For this review, use the dimensioned drawing (mm, ordinates from the lowest corner) and the shaded views. Coordinates: 2 decimals unless noted, no trailing zeros. Loops run counter-clockwise (first coordinate to the right, second up) from the corner with the lowest first, then second, coordinate; pieces in that order, holes last. Notation, with made-up numbers: (86, 82) - (100, 82) arc R28 cw to (100, 112) - close; hole circle Ø4 at (20.25, 70). An arc over 180 degrees is marked (long way). Answer in a Markdown table with one row per item. Add a question column.
(1) We need section B-B, the plane z = 22.5. Write out the cut boundary in (x, y), plus the area to 3 significant figures.
(2) To check wall thickness, follow L1, parallel to Y at x = 24, z = 10.5; L2, parallel to Y at x = 23.5, z = 1.5; L3, parallel to Z at x = 11.5, y = 41. State the ranges of each line that lie inside material, in increasing order. Write a range as [from, to].
(3) Clearance check with flat-ended pins moving along their axes: pin 1 (9 mm diameter, centred on x = 24, y = 24, fed in from -Z); pin 2 (1.5 mm diameter, centred on x = 18.5, z = 4.5, fed in from +Y); pin 3 (5 mm diameter, centred on y = 13, z = 13, fed in from -X); pin 4 (3 mm diameter, centred on x = 31.5, z = 7, fed in from +Y). State where each tip first meets the part, or that it passes through.
(4) The part is to be moulded in two halves that separate along Y. For the marked faces 1, 2 and 3, say which applies: released by +Y, released by -Y, zero draft, split by the parting line, or undercut.
(5) We need section A-A, the plane z = 6.25. Write out the cut boundary in (x, y).
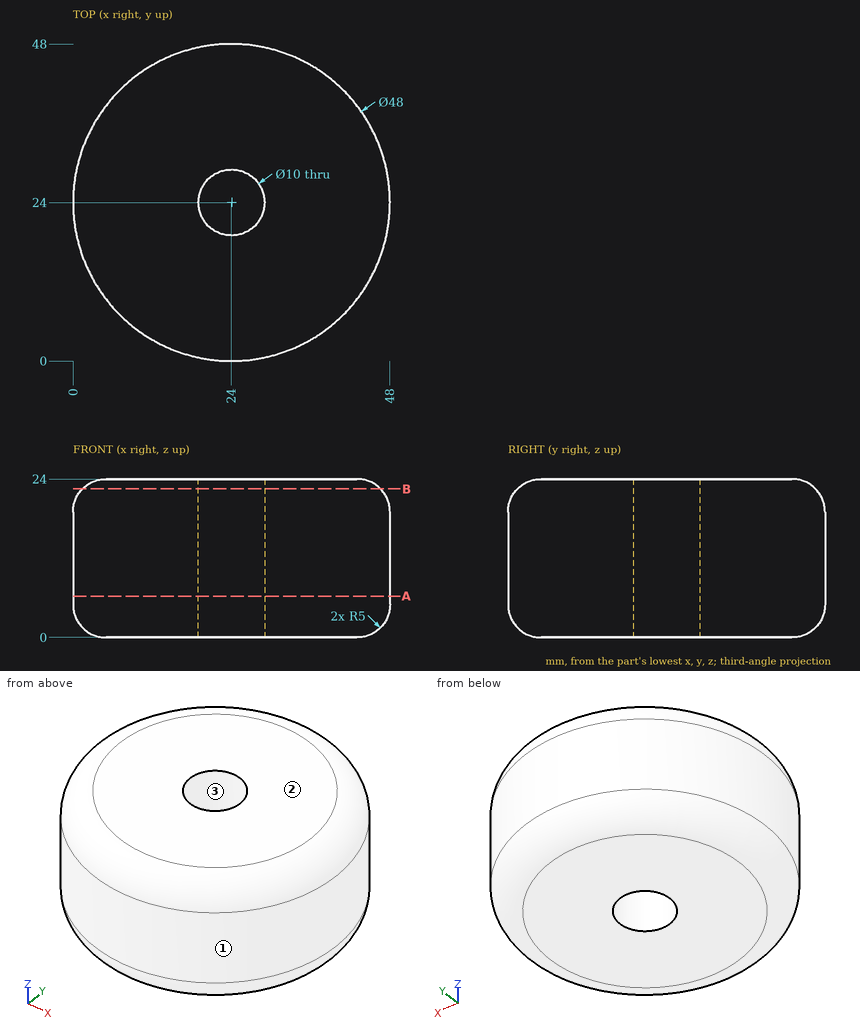
Responses:
| question | item | result |
|---|---|---|
| 1 | outline | circle Ø45.14 at (24, 24); hole circle Ø10 at (24, 24) |
| 1 | area | 1,520 mm2 |
| 2 | L1 | y = [0, 19], [29, 48] |
| 2 | L2 | y = [1.43, 19.03], [28.97, 46.57] |
| 2 | L3 | z = [0.46, 23.54] |
| 3 | pin 1 | passes through |
| 3 | pin 2 | stops at y = 47.51 |
| 3 | pin 3 | stops at x = 1.56 |
| 3 | pin 4 | stops at y = 47.24 |
| 4 | face 1 | split by the parting line |
| 4 | face 2 | zero draft |
| 4 | face 3 | undercut |
| 5 | outline | circle Ø48 at (24, 24); hole circle Ø10 at (24, 24) |
